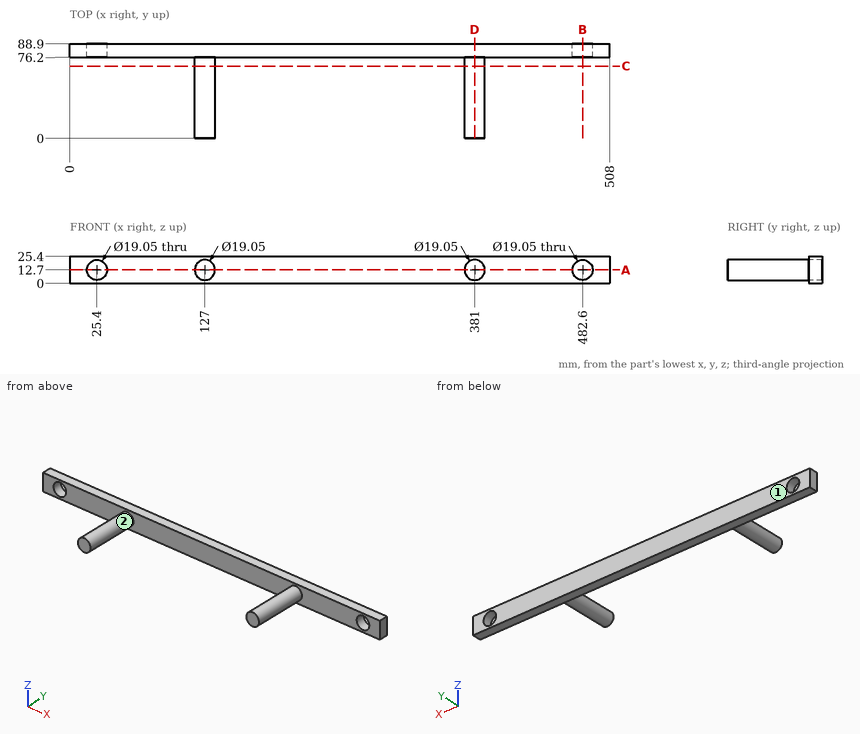
For this review, use the dimensioned drawing (mm, ordinates from the lowest corner) and the shaded views. Coordinates: 2 decimals unless noted, no trailing zeros. Loops run counter-clockwise (first coordinate to the right, second up) from the corner with the lowest first, then second, coordinate; pieces in that order, holes last. Notation, with made-up numbers: (-37, 41.5) -> (-28, 41.5) arc R28 cw to (-28, 69.5) -> close; hole circle Ø2 at (34.25, 89). An arc over 180 degrees is marked (long way). Return JSON: item names as keys, results as strings. Group by question number.
(1) Consider section C-C, the plane y = 68. Give the boundary of the cut face in (x, z) (3 decimals).
(2) Consider section B-B, the plane x = 482.6. Give the boundary of the cut face in (y, z) (3 decimals).
(3) Mouldability with a two-part tool opening along X and no side actions: class the marked faces 1 and 2 as pulls with the +X half, pulls with the -X half, needs draft (parallel to the pull), parting line crosses it, or undercut.
(4) Consider section A-A, the plane z = 12.7. Give the boundary of the cut face in (x, y) (3 decimals), plus the area to 3 significant figures.
(5) Consider section D-D, the plane x = 381. Give the boundary of the cut face in (y, z) (3 decimals), plus the area to 3 significant figures.
(6) For pin 1 Ø10 at (y, z) = (42, 17.5) entering from -X (3 decimals); pin 2 Ø1.5 at (y, z) = (15, 9) entering from +X; pin 3 Ø3 at (y, z) = (30, 8.5) entering from -X; pin 4 Ø15 at (x, z) = (482.6, 12.7) entering from -Y, all flat-tipped, find the tip position at first contact; note any pin that passes through.
(7) To check wall thickness, follow L1, parallel to X at y = 85, z = 12.7 (3 decimals); L2, parallel to Z at x = 482, y = 81; L3, parallel to X at y = 75.5, z = 13.5. State the ranges of each line that lie inside material, in increasing order.
Results below:
{
 "1": {"outline": "circle Ø19.05 at (127, 12.7); circle Ø19.05 at (381, 12.7)"},
 "2": {"outline": "(76.2, 0) -> (88.9, 0) -> (88.9, 3.175) -> (76.2, 3.175) -> close; (76.2, 22.225) -> (88.9, 22.225) -> (88.9, 25.4) -> (76.2, 25.4) -> close"},
 "3": {"face 1": "needs draft", "face 2": "undercut"},
 "4": {"outline": "(0, 76.2) -> (15.875, 76.2) -> (15.875, 88.9) -> (0, 88.9) -> close; (34.925, 76.2) -> (117.475, 76.2) -> (117.475, 0) -> (136.525, 0) -> (136.525, 76.2) -> (371.475, 76.2) -> (371.475, 0) -> (390.525, 0) -> (390.525, 76.2) -> (473.075, 76.2) -> (473.075, 88.9) -> (34.925, 88.9) -> close; (492.125, 76.2) -> (508, 76.2) -> (508, 88.9) -> (492.125, 88.9) -> close", "area": "8,870 mm2"},
 "5": {"outline": "(0, 3.175) -> (76.2, 3.175) -> (76.2, 0) -> (88.9, 0) -> (88.9, 25.4) -> (76.2, 25.4) -> (76.2, 22.225) -> (0, 22.225) -> close", "area": "1,770 mm2"},
 "6": {"pin 1": "stops at x = 117.475", "pin 2": "stops at x = 390.06", "pin 3": "stops at x = 117.87", "pin 4": "passes through"},
 "7": {"L1": "x = 0 to 15.875, 34.925 to 473.075, 492.125 to 508", "L2": "z = 0 to 3.19, 22.21 to 25.4", "L3": "x = 117.51 to 136.49, 371.51 to 390.49"}
}
